Geometry check sheet. Reference: the model listing, model coordinates, mm. Coordinates: 2 decimals unless noted, no trailing zeros. Write each loop counter-clockwise with the first axis right and the second up, starting at its lowest first coordinate (ties: lowest second). Pieces come first, ordered by that corner, then holes. Notation, with made-up numbers: (59.5, 45.5) -> (73.5, 45.5) arc R11 ccw to (73.5, 54.5) -> close; hole circle Ø2 at (33.25, 54). An arc over 180 degrees is marked (long way). Answer in a Markdown table with one row per item. Add a question column.
1. Cross-section at A-A on y = 57.5. Record the cut outline in (x, z).
2. Depth check by flat-ended pin: P1, Ø5, axis at x = 0, y = -189.97, coming from the +Z side; P2, Ø3, axis at x = 0, y = -37.5, coming from the -Z side. Enter the tip coordinate at first touch or a pass-through.
3. Cross-section at B-B on x = 0. Give the number of separate pieces and of enclosed holes in the cut face, and give its area (3 significant figures).
4. Scan lines: L1, parallel to X at y = 209.97, z = 4.3; L2, parallel to X at y = 99, z = 0.25. Record each from-to range of solid material in increasing order. Write a range as from..to.
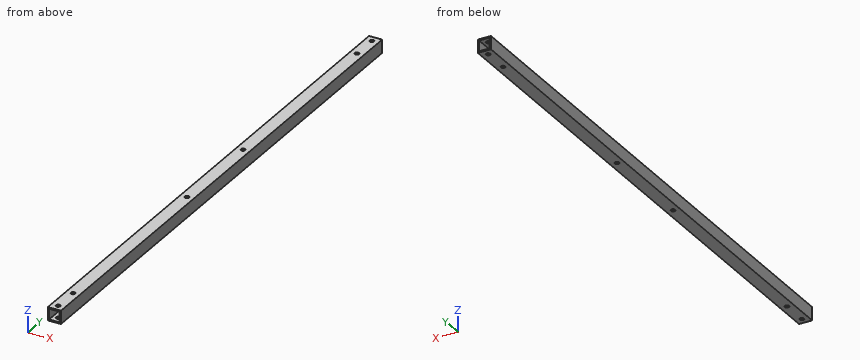
```python
from build123d import *

# Parameters (mm, degrees)
SKETCH_1_W          = 10
SKETCH_1_H          = 10
SKETCH_1_W_2        = 8
SKETCH_1_H_2        = 8
EXTRUDE_1_DEPTH     = 214.97
SKETCH_2_R          = 1.6
CUT_EXTRUDE_1_DEPTH = 213.715
SKETCH_3_R          = 1.6
CUT_EXTRUDE_2_DEPTH = 10


with BuildPart() as part:
    # ｽｹｯﾁ1 → ﾎﾞｽ - 押し出し1 (new, symmetric)
    with BuildSketch(Plane(origin=(0, 0, 0), x_dir=(1, 0, 0), z_dir=(0, 1, 0))):
        Rectangle(SKETCH_1_W, SKETCH_1_H)
        Rectangle(SKETCH_1_W_2, SKETCH_1_H_2, mode=Mode.SUBTRACT)
    extrude(amount=EXTRUDE_1_DEPTH, both=True)

    # ｽｹｯﾁ2 → ｶｯﾄ - 押し出し1 (cut, symmetric)
    with BuildSketch(Plane.XY.offset(5)):
        with Locations((0, 209.97)):
            Circle(SKETCH_2_R)
        with Locations((0, 189.97)):
            Circle(SKETCH_2_R)
    cut_extrude_1 = extrude(amount=CUT_EXTRUDE_1_DEPTH, both=True, mode=Mode.SUBTRACT)

    # ﾐﾗｰ1: ｶｯﾄ - 押し出し1 across plane
    add(cut_extrude_1.mirror(Plane.ZX), mode=Mode.SUBTRACT)

    # ｽｹｯﾁ3 → ｶｯﾄ - 押し出し2 (cut)
    with BuildSketch(Plane(origin=(0, 0, -5), x_dir=(-1, 0, 0), z_dir=(0, 0, -1))):
        with Locations((0, 37.5)):
            Circle(SKETCH_3_R)
        with Locations((0, -37.5)):
            Circle(SKETCH_3_R)
    extrude(amount=-CUT_EXTRUDE_2_DEPTH, mode=Mode.SUBTRACT)


solid = part.part
```
Results found:
| question | item | result |
|---|---|---|
| 1 | outline | (-5, -5) -> (5, -5) -> (5, 5) -> (-5, 5) -> close; hole (-4, -4) -> (4, -4) -> (4, 4) -> (-4, 4) -> close |
| 2 | P1 | stops at z = 5 |
| 2 | P2 | passes through |
| 3 | separate pieces | 14 |
| 3 | enclosed holes | 0 |
| 3 | area | 821 mm^2 |
| 4 | L1 | x = -5..-1.6, 1.6..5 |
| 4 | L2 | x = -5..-4, 4..5 |
